Here's how the part is built. I have some questions about the finished solid (model axes, mm). Round coordinates to 2 decimals unless told otherwise and drop trailing zeros. Loops run counter-clockwise (first coordinate to the right, second up) from the corner with the lowest first, then second, coordinate; pieces in that order, holes last. Notation, with made-up numbers: M 25,82 L 78,82 A33 cw 78,120 Z; hole C -25.5,-39 d11. An arc over 180 degrees is marked long. Use a Markdown table: item, result.
Autodesk Inventor part; units mm, degrees
ref_plane "YZ Plane" through (0, 0, 0) normal (1, 0, 0) x (0, 1, 0)
ref_plane "XZ Plane" through (0, 0, 0) normal (0, 1, 0) x (-1, 0, 0)
ref_plane "XY Plane" through (0, 0, 0) normal (0, 0, 1) x (1, 0, 0)
sketch "Sketch1" plane through (0, 0, 0) normal (0, 1, 0) x (-1, 0, 0)
  circle A0 centre (0, 0) radius 20
  dimension "d0" = 40
extrude "Extrusion1" add sketch "Sketch1" along normal blind 2.6
sketch "Sketch2" plane through (0, 2.6, 0) normal (0, 1, 0) x (1, 0, 0)
  line L0 (-10, -10) -> (-10, 10)
  line L1 (-10, 10) -> (10, 10)
  line L2 (10, 10) -> (10, -10)
  line L3 (10, -10) -> (-10, -10)
  line L4 (-10, -10) -> (10, 10) construction
  line L5 (-10, 10) -> (10, -10) construction
  point P0 (0, 0)
  dimension "d3" = 20
  dimension "d4" = 20
extrude "Extrusion2" cut sketch "Sketch2" against normal blind 0.6
sketch "Sketch3" plane through (0, 2, 0) normal (0, 1, 0) x (1, 0, 0)
  line L0 (-6.3669, 8.3364) -> (6.4396, 8.3364) construction
  line L1 (6.4396, 8.3364) -> (6.4396, -8.2636) construction
  line L2 (6.4396, -8.2636) -> (-6.3669, -8.2636) construction
  line L3 (-6.3669, -8.2636) -> (-6.3669, 8.3364) construction
  line L4 (-4.6854, -8.2636) -> (-4.6854, 8.3364)
  line L5 (-4.6854, 8.3364) -> (5.6997, 8.3364)
  line L6 (5.6997, 8.3364) -> (5.6997, 6.3723)
  line L7 (5.6997, 6.3723) -> (-2.4792, 6.3723)
  line L8 (-2.4792, 6.3723) -> (-2.4792, 1.8255)
  line L9 (-2.4792, 1.8255) -> (5.1482, 1.8255)
  line L10 (5.1482, 1.8255) -> (5.1482, -0.1385)
  line L11 (5.1482, -0.1385) -> (-2.4792, -0.1385)
  line L12 (-2.4792, -0.1385) -> (-2.4792, -6.2996)
  line L13 (-2.4792, -6.2996) -> (5.6997, -6.2996)
  line L14 (5.6997, -6.2996) -> (5.6997, -8.2636)
  line L15 (5.6997, -8.2636) -> (-4.6854, -8.2636)
  point P0 (0, 0)
extrude "Extrusion3" add sketch "Sketch3" along normal blind 0.6
properties part number "TopMarkerPreset"
1. For pin 1 Ø0.5 at (y, z) = (2.5, -3) entering from -X; pin 2 Ø1.5 at (y, z) = (1.5, 1.5) entering from -X; pin 3 Ø0.7 at (x, y) = (-0.5, 2.5) entering from +Z, each with a flat end and sliding along its axis, tell me the tip position at first contact or that it passes through.
Answer sheet:
| item | result |
|---|---|
| pin 1 | x = -19.81 |
| pin 2 | x = -19.99 |
| pin 3 | z = 20 |
2. Imagine slicing it at D-D, the plane z = 12. Write out the boundary of the cut face in (x, y), then the cut area to 3 significant figures.
Answer sheet:
| item | result |
|---|---|
| outline | M -16,0 L 16,0 L 16,2.6 L -16,2.6 Z |
| area | 83.2 mm2 |
3. Imagine slicing it at C-C, the plane y = 0.7. Write out the boundary of the cut face in (x, z).
Answer sheet:
| item | result |
|---|---|
| outline | C 0,0 d40 |
4. Imagine slicing it at A-A, the plane z = -7.5. Write out the boundary of the cut face in (x, y), then the cut area to 3 significant figures.
Answer sheet:
| item | result |
|---|---|
| outline | M -18.54,0 L 18.54,0 L 18.54,2.6 L 10,2.6 L 10,2 L 5.7,2 L 5.7,2.6 L -4.69,2.6 L -4.69,2 L -10,2 L -10,2.6 L -18.54,2.6 Z |
| area | 90.6 mm2 |
5. We'd pull the mould along X, two halves only. Please class faces 1 (the face through (0, 2, -2)), 2 (the face through (4.336, 1.282, 19.524)), 3 (the face through (-13, 2.6, 0)): +X half, -X half, draft (parallel to the pull), parting line (faces both ways), or undercut.
Answer sheet:
| item | result |
|---|---|
| face 1 | undercut |
| face 2 | parting line |
| face 3 | draft |
6. I need wall thicknesses on probe 1 along X at (y, z) = (2.35, 1.5); probe 2 along X at (y, z) = (2.25, -8); probe 3 along X at (y, z) = (0.7, 0.5). Which ranges of each line are inside material? Lowest first, please. Write a range as from..to.
Answer sheet:
| item | result |
|---|---|
| probe 1 | -19.94..-10, -4.69..-2.48, 10..19.94 |
| probe 2 | -18.33..-10, -4.69..5.7, 10..18.33 |
| probe 3 | -19.99..19.99 |
7. Imagine slicing it at B-B, the plane x = 0. Write out the boundary of the cut face in (y, z).
Answer sheet:
| item | result |
|---|---|
| outline | M 0,-20 L 2.6,-20 L 2.6,-10 L 2,-10 L 2,-8.34 L 2.6,-8.34 L 2.6,-6.37 L 2,-6.37 L 2,-1.83 L 2.6,-1.83 L 2.6,0.14 L 2,0.14 L 2,6.3 L 2.6,6.3 L 2.6,8.26 L 2,8.26 L 2,10 L 2.6,10 L 2.6,20 L 0,20 Z |
